CAD build for the part. Positions are in the model's coordinates, mm. Face numbers are marked on the shaded views. Round coordinates to 2 decimals unless told otherwise and drop trailing zeros. Loops run counter-clockwise (first coordinate to the right, second up) from the corner with the lowest first, then second, coordinate; pieces in that order, holes last. Notation, with made-up numbers: (15, -21) - (53, -21) arc R21 ccw to (53, 5) - close; hole circle Ø3 at (10, 13). An arc over 180 degrees is marked (long way). One line per question, with ' | ' between items.
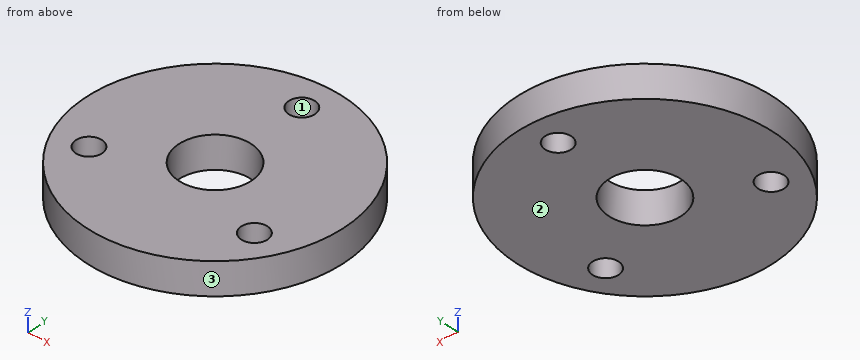
```python
from build123d import *

# Parameters (mm, degrees)
SKETCH1_R           = 25.4
BOSS_EXTRUDE1_DEPTH = 6.35
SKETCH1_3_R         = 2.5781
CUT_EXTRUDE1_DEPTH  = 6.35
SKETCH1_5_R         = 7.1501
CUT_EXTRUDE2_DEPTH  = 6.35


with BuildPart() as part:
    # Sketch1 → Boss-Extrude1 (new body)
    with BuildSketch(Plane.XY):
        Circle(SKETCH1_R)
    extrude(amount=BOSS_EXTRUDE1_DEPTH)

    # Sketch1<3> → Cut-Extrude1 (cut)
    with BuildSketch(Plane.XY):
        with Locations((0, 19.05)):
            Circle(SKETCH1_3_R)
        with Locations((16.497783942, -9.525)):
            Circle(SKETCH1_3_R)
        with Locations((-16.497783942, -9.525)):
            Circle(SKETCH1_3_R)
    extrude(amount=CUT_EXTRUDE1_DEPTH, mode=Mode.SUBTRACT)

    # Sketch1<5> → Cut-Extrude2 (cut)
    with BuildSketch(Plane.XY):
        Circle(SKETCH1_5_R)
    extrude(amount=CUT_EXTRUDE2_DEPTH, mode=Mode.SUBTRACT)


solid = part.part
```
(1) Cut at B-B, the plane x = 17. Write the cut outline in (y, z).
Results found:
outline: (-18.87, 0) - (-12.05, 0) - (-12.05, 6.35) - (-18.87, 6.35) - close; (-7, 0) - (18.87, 0) - (18.87, 6.35) - (-7, 6.35) - close
(2) Cut at D-D, the plane z = 1.25. Write the cut outline in (x, y) (3 decimals), then the cut area to 3 significant figures.
Results found:
outline: circle Ø50.8 at (0, 0); hole circle Ø5.156 at (-16.498, -9.525); hole circle Ø14.3 at (0, 0); hole circle Ø5.156 at (0, 19.05); hole circle Ø5.156 at (16.498, -9.525) | area: 1,800 mm²
(3) Cut at A-A, the plane y = 0. Write the cut outline in (x, z).
Results found:
outline: (-25.4, 0) - (-7.15, 0) - (-7.15, 6.35) - (-25.4, 6.35) - close; (7.15, 0) - (25.4, 0) - (25.4, 6.35) - (7.15, 6.35) - close
(4) Drop a flat-ended pin along its axis: P1, Ø4.5, axis at x = 16.5, y = -9.52, coming from the +Z side. Give the stop position or say it passes through.
Results found:
P1: passes through
(5) Two-plate mould, pull along Y, no slides. Class the marked faces 1, 2 and 3: released by +Y, released by -Y, zero draft, split by the parting line, or undercut.
Results found:
face 1: undercut | face 2: zero draft | face 3: split by the parting line
(6) Probe L1, parallel to Y at x = 0, z = 4.5; L2, parallel to X at y = -11.5, z = 5; L3, parallel to X at y = 21, z = 1.75. List the from-to ranges inside material, lowest first.
Results found:
L1: y = -25.4 to -7.15, 7.15 to 16.47, 21.63 to 25.4 | L2: x = -22.65 to -18.15, -14.84 to 14.84, 18.15 to 22.65 | L3: x = -14.29 to -1.69, 1.69 to 14.29
(7) Cut at C-C, the plane x = 0. Write the cut outline in (y, z), then the cut area to 3 significant figures.
Results found:
outline: (-25.4, 0) - (-7.15, 0) - (-7.15, 6.35) - (-25.4, 6.35) - close; (7.15, 0) - (16.47, 0) - (16.47, 6.35) - (7.15, 6.35) - close; (21.63, 0) - (25.4, 0) - (25.4, 6.35) - (21.63, 6.35) - close | area: 199 mm²
